Geometry: final body of the model. Coordinates: model frame, mm. A direction names the side the tool comes from. Round coordinates to 2 decimals unless told otherwise and drop trailing zeros. Loops run counter-clockwise (first coordinate to the right, second up) from the corner with the lowest first, then second, coordinate; pieces in that order, holes last. Notation, with made-up numbers: (-29.5, 69) -> (9.5, 69) arc R19 ccw to (9.5, 104) -> close; hole circle Ø4 at (1, -39.75). An arc over 180 degrees is marked (long way). Answer in a Markdown table with one row per item.
```python
from build123d import *

# Parameters (mm, degrees)
SKETCH1_R           = 2.5
EXTRUDE_1_DEPTH     = 220
SKETCH_1_R          = 1.7
CUT_EXTRUDE_1_DEPTH = 221.665380157


with BuildPart() as part:
    # Sketch1 → 凸台-拉伸1 (new body)
    with BuildSketch(Plane.XY):
        with BuildLine():
            Line((-3.6, 10), (-3.6, 9.5))
            Line((-3.6, 9.5), (-3.1, 9.5))
            Line((-3.1, 9.5), (-3.1, 8.5))
            Line((-3.1, 8.5), (-5.5, 8.5))
            Line((-5.5, 8.5), (-5.5, 6.65))
            Line((-5.5, 6.65), (-2.75, 3.9))
            Line((-2.75, 3.9), (2.75, 3.9))
            Line((2.75, 3.9), (5.5, 6.65))
            Line((5.5, 6.65), (5.5, 8.5))
            Line((5.5, 8.5), (3.1, 8.5))
            Line((3.1, 8.5), (3.1, 9.5))
            Line((3.1, 9.5), (3.6, 9.5))
            Line((3.6, 9.5), (3.6, 10))
            Line((3.6, 10), (8.5, 10))
            ThreePointArc((8.5, 10), (9.560660172, 9.560660172), (10, 8.5))
            Line((10, 8.5), (10, 3.6))
            Line((10, 3.6), (9.5, 3.6))
            Line((9.5, 3.6), (9.5, 3.1))
            Line((9.5, 3.1), (8.5, 3.1))
            Line((8.5, 3.1), (8.5, 5.5))
            Line((8.5, 5.5), (6.65, 5.5))
            Line((6.65, 5.5), (3.9, 2.75))
            Line((3.9, 2.75), (3.9, -2.75))
            Line((3.9, -2.75), (6.65, -5.5))
            Line((6.65, -5.5), (8.5, -5.5))
            Line((8.5, -5.5), (8.5, -3.1))
            Line((8.5, -3.1), (9.5, -3.1))
            Line((9.5, -3.1), (9.5, -3.6))
            Line((9.5, -3.6), (10, -3.6))
            Line((10, -3.6), (10, -8.5))
            ThreePointArc((10, -8.5), (9.560660172, -9.560660172), (8.5, -10))
            Line((8.5, -10), (3.6, -10))
            Line((3.6, -10), (3.6, -9.5))
            Line((3.6, -9.5), (3.1, -9.5))
            Line((3.1, -9.5), (3.1, -8.5))
            Line((3.1, -8.5), (5.5, -8.5))
            Line((5.5, -8.5), (5.5, -6.65))
            Line((5.5, -6.65), (2.75, -3.9))
            Line((2.75, -3.9), (-2.75, -3.9))
            Line((-2.75, -3.9), (-5.5, -6.65))
            Line((-5.5, -6.65), (-5.5, -8.5))
            Line((-5.5, -8.5), (-3.1, -8.5))
            Line((-3.1, -8.5), (-3.1, -9.5))
            Line((-3.1, -9.5), (-3.6, -9.5))
            Line((-3.6, -9.5), (-3.6, -10))
            Line((-3.6, -10), (-8.5, -10))
            ThreePointArc((-8.5, -10), (-9.560660172, -9.560660172), (-10, -8.5))
            Line((-10, -8.5), (-10, -3.6))
            Line((-10, -3.6), (-9.5, -3.6))
            Line((-9.5, -3.6), (-9.5, -3.1))
            Line((-9.5, -3.1), (-8.5, -3.1))
            Line((-8.5, -3.1), (-8.5, -5.5))
            Line((-8.5, -5.5), (-6.65, -5.5))
            Line((-6.65, -5.5), (-3.9, -2.75))
            Line((-3.9, -2.75), (-3.9, 2.75))
            Line((-3.9, 2.75), (-6.65, 5.5))
            Line((-6.65, 5.5), (-8.5, 5.5))
            Line((-8.5, 5.5), (-8.5, 3.1))
            Line((-8.5, 3.1), (-9.5, 3.1))
            Line((-9.5, 3.1), (-9.5, 3.6))
            Line((-9.5, 3.6), (-10, 3.6))
            Line((-10, 3.6), (-10, 8.5))
            ThreePointArc((-10, 8.5), (-9.560660172, 9.560660172), (-8.5, 10))
            Line((-8.5, 10), (-3.6, 10))
        make_face()
        Circle(SKETCH1_R, mode=Mode.SUBTRACT)
    extrude(amount=EXTRUDE_1_DEPTH)

    # 草图1 → 切除-拉伸1 (cut, through all)
    with BuildSketch(Plane(origin=(0, 3.9, 0), x_dir=(1, 0, 0), z_dir=(0, 1, 0))):
        with Locations(Location((0, -214, 0), (0, 0, 180))):
            Circle(SKETCH_1_R)
        with Locations(Location((0, -6, 0), (0, 0, 180))):
            Circle(SKETCH_1_R)
    extrude(amount=-CUT_EXTRUDE_1_DEPTH, mode=Mode.SUBTRACT)


solid = part.part
```
Item 1: Set-up query: faces 5 (the cylindrical face through (-1.57, 3.11, 213.35)), 6 (the flat face through (0, -3.9, 108)), 7 (the flat face through (0, 3.9, 108)). Return all of +Z, -Z, +X, -X, +Y, -Y with unobstructed straight access to the full face (end or side cutting, diameter ignored); none if empty.
Ans:
| item | result |
|---|---|
| face 5 | +Y, -Y |
| face 6 | +Z, -Z, -Y |
| face 7 | +Z, -Z, +Y |
Item 2: Ray query, L1, parallel to Z at x = 0, y = -3.1; L2, parallel to Y at x = 8, z = 55.5; L3, parallel to Y at x = 0, z = 121.5. Return the intervals inside material, ascending.
Ans:
| item | result |
|---|---|
| L1 | 0 to 4.3, 7.7 to 212.3, 215.7 to 220 |
| L2 | -10 to -5.5, 5.5 to 10 |
| L3 | -3.9 to -2.5, 2.5 to 3.9 |
Item 3: First-contact query: P1, Ø3, axis at y = 1, z = 77, coming from the +X side; P2, Ø0.8, axis at x = -9, z = 162, coming from the +Y side; P3, Ø0.6, axis at y = -9.5, z = 116.5, coming from the +X side. Flat tips, straight axial feed; report the tip coordinate or a pass-through.
Ans:
| item | result |
|---|---|
| P1 | x = 3.9 |
| P2 | y = 10 |
| P3 | x = 9.83 |
Item 4: Section query A-A, the plane y = 0. Output: boundary loops of the cut face in (x, z), and give its area (3 significant figures).
Ans:
| item | result |
|---|---|
| outline | (-3.9, 0) -> (-2.5, 0) -> (-2.5, 220) -> (-3.9, 220) -> close; (2.5, 0) -> (3.9, 0) -> (3.9, 220) -> (2.5, 220) -> close |
| area | 616 mm2 |
Item 5: Mould query, pull axis Y, two halves, no side actions, for faces 1 (the flat face through (3.9, 0, 108)), 2 (the flat face through (6, 10, 108)), 3 (the flat face through (10, 6, 108)), 4 (the cylindrical face through (-0.54, -2.44, 108.46)). Classes: released by +Y, released by -Y, zero draft, split by the parting line, or undercut.
Ans:
| item | result |
|---|---|
| face 1 | undercut |
| face 2 | released by +Y |
| face 3 | zero draft |
| face 4 | undercut |
